```python
from build123d import *

# Parameters (mm, degrees)
F0_R          = 0.5
F1_DEPTH      = 10
F0_R_2        = 0.75
F2_DEPTH      = 0.5
F3_R          = 0.1
F5_DEPTH      = 25
F5_DEPTH_BACK = 25


with BuildPart() as f1:
    # F0 (on Top) → F1 (new body)
    with BuildSketch(Plane.XY):
        Circle(F0_R)
    extrude(amount=F1_DEPTH)

    # F0 (on Top) → F2 (join)
    with BuildSketch(Plane.XY):
        Circle(F0_R_2)
        Circle(F0_R, mode=Mode.SUBTRACT)
    extrude(amount=F2_DEPTH)

    # F3
    f3_edges = [f1.edges().sort_by_distance(p)[0] for p in [
        (-0.75, 0, 0),
    ]]
    fillet(f3_edges, radius=F3_R)

    # F4 (on Front) → F5 (cut, two sides)
    with BuildSketch(Plane.XZ) as f5_sk:
        Polygon((-0.6920135929, 8.791741915), (0, 10.0138969719), (0.6348980824, 8.791741915), (0.6348980824, 10.8100445941), (-0.7408999372, 10.8100445941), (-0.7408999372, 8.791741915), align=None)
    extrude(amount=-F5_DEPTH, mode=Mode.SUBTRACT)
    extrude(f5_sk.sketch, amount=F5_DEPTH_BACK, mode=Mode.SUBTRACT)


solid = f1.part
```
The listing builds one solid part. Answer for the finished solid, in the listing's coordinates (mm). A direction names the side the tool comes from. Give positions to 0.01 mm unless a question says otherwise; leave off trailing zeros. Order: outer loops, then holes, each group sorted by start corner. A loop starts at its lowest first (then second) coordinate and runs counter-clockwise, first axis right, second up.
Item 1: Which of the six approach directions +Z, -Z, +X, -X, +Y, -Y give full straight-line access (tool end or side, diameter ignored) to faces 1 (the face through (0.195, 0.007, 9.638)), 2 (the face through (0.462, -0.192, 5.184))?
From the geometry:
face 1: +Z, +X, +Y, -Y
face 2: +Z
Item 2: Find the intervals of material crossed by probe 1 along Z at (x, y) = (-0.5, 0.45); probe 2 along X at (y, z) = (0, 5.5), in increasing order.
From the geometry:
probe 1: z = 0 to 0.5
probe 2: x = -0.5 to 0.5
Item 3: The part is cut by section C-C, the plane z = 9.75. Give the vertices of the cut face in (x, y).
From the geometry:
outline: (-0.15, -0.48) arc R0.5 ccw to (0.14, -0.48) - (0.14, 0.48) arc R0.5 ccw to (-0.15, 0.48) - close
Item 4: The part is cut by section B-B, the plane z = 4.5. Give the vertices of the cut face in (x, y).
From the geometry:
outline: circle Ø1 at (0, 0)
